Source: CAD feature listing. Evaluate the final solid. Frame: model axes, mm. Face numbers are marked on the shaded views. A direction names the side the tool comes from. Round coordinates to 2 decimals unless told otherwise and drop trailing zeros. Loops run counter-clockwise (first coordinate to the right, second up) from the corner with the lowest first, then second, coordinate; pieces in that order, holes last. Notation, with made-up numbers: M 21,44.5 L 30,44.5 A10 ccw 30,63.5 Z; hole C 43,8 d11. An arc over 180 degrees is marked long. Write each question's results on one line, items separated by ' | '. Start each with the question number.
1. Section A-A on x = -1.5. Output: boundary loops of the cut face in (y, z), and give its area (3 significant figures).
2. Section B-B on z = 7.5. Output: boundary loops of the cut face in (x, y).
3. Section D-D on y = -33.5. Output: boundary loops of the cut face in (x, z), and give its area (3 significant figures).
4. Section C-C on y = -7. Output: boundary loops of the cut face in (x, z), and give its area (3 significant figures).
5. Contact query for a flat-ended pin moving along its axis: pin 1 Ø1.6 at (x, z) = (12.5, -1.5) entering from -Y. Output: stop coordinate, or through.
6. Ray query, line 1 (X direction, y = -25, z = 17); line 2 (Z direction, x = 1, y = -25); line 3 (X direction, y = -21.5, z = -3). Return the intervals inside material, ascending.
7. Draft query along Z for the marked faces 1, 2 and 3. Return one class per face: released by +Z, released by -Z, zero draft, split by the parting line, or undercut.
8. Set-up query: the marked faces 4 and 5. Return all of +Z, -Z, +X, -X, +Y, -Y with unobstructed straight access to the full face (end or side cutting, diameter ignored); none if empty.
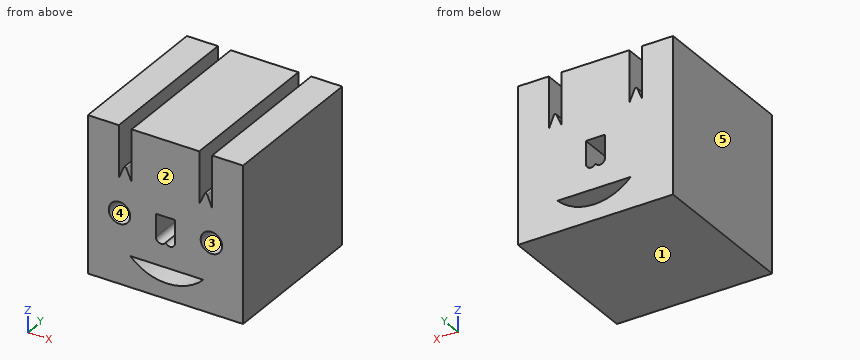
from build123d import *

# Parameters (mm, degrees)
F0_R     = 2.637924
F1_DEPTH = 38.1
F2_DEPTH = 19.05


with BuildPart() as f1:
    # F0 (on Front) → F1 (new body)
    with BuildSketch(Plane.XZ):
        with BuildLine():
            Line((-11.453714, 19.05), (-19.05, 19.05))
            Line((-19.05, 19.05), (-19.05, -19.05))
            Line((-19.05, -19.05), (19.05, -19.05))
            Line((19.05, -19.05), (19.05, 19.05))
            Line((19.05, 19.05), (11.453714, 19.05))
            Line((11.453714, 19.05), (11.453714, 6.35))
            Line((11.453714, 6.35), (10.227945, 9.297051))
            ThreePointArc((10.227945, 9.297051), (9.928561, 9.499715), (9.623805, 9.305221))
            Line((9.623805, 9.305221), (8.299793, 6.35))
            Line((8.299793, 6.35), (8.299793, 19.05))
            Line((8.299793, 19.05), (0, 19.05))
            Line((0, 19.05), (-8.299793, 19.05))
            Line((-8.299793, 19.05), (-8.299793, 6.35))
            Line((-8.299793, 6.35), (-9.623805, 9.305221))
            ThreePointArc((-9.623805, 9.305221), (-9.928561, 9.499715), (-10.227945, 9.297051))
            Line((-10.227945, 9.297051), (-11.453714, 6.35))
            Line((-11.453714, 6.35), (-11.453714, 19.05))
        make_face()
        with Locations((-11.287717, -1.99195)):
            Circle(F0_R, mode=Mode.SUBTRACT)
        with BuildLine():
            ThreePointArc((9.332039, -11.526389), (0.341904, -15.257474), (-8.648231, -11.526389))
            Line((-8.648231, -11.526389), (9.332039, -11.526389))
        make_face(mode=Mode.SUBTRACT)
        with BuildLine():
            Line((-2.361556, 0.645974), (0, 0.645974))
            Line((0, 0.645974), (2.361556, 0.645974))
            Line((2.361556, 0.645974), (2.361556, -4.915977))
            ThreePointArc((2.361556, -4.915977), (1.428174, -6.140554), (0, -5.565134))
            ThreePointArc((0, -5.565134), (-1.428174, -6.140554), (-2.361556, -4.915977))
            Line((-2.361556, -4.915977), (-2.361556, 0.645974))
        make_face(mode=Mode.SUBTRACT)
        with Locations((11.287717, -1.99195)):
            Circle(F0_R, mode=Mode.SUBTRACT)
    extrude(amount=F1_DEPTH)

    # F0 (on Front) → F2 (join)
    with BuildSketch(Plane.XZ):
        with Locations((-11.287717, -1.99195)):
            Circle(F0_R)
        with Locations((11.287717, -1.99195)):
            Circle(F0_R)
    extrude(amount=F2_DEPTH)


solid = f1.part
Taken from the geometry:
1) outline: M -38.1,-19.05 L 0,-19.05 L 0,-15.12 L -38.1,-15.12 Z; M -38.1,-11.53 L 0,-11.53 L 0,-6.12 L -38.1,-6.12 Z; M -38.1,0.65 L 0,0.65 L 0,19.05 L -38.1,19.05 Z | area: 1,060 mm^2
2) outline: M -19.05,-38.1 L -11.45,-38.1 L -11.45,0 L -19.05,0 Z; M -10.98,-38.1 L -8.82,-38.1 L -8.82,0 L -10.98,0 Z; M -8.3,-38.1 L 8.3,-38.1 L 8.3,0 L -8.3,0 Z; M 8.82,-38.1 L 10.98,-38.1 L 10.98,0 L 8.82,0 Z; M 11.45,-38.1 L 19.05,-38.1 L 19.05,0 L 11.45,0 Z
3) outline: M -19.05,-19.05 L 19.05,-19.05 L 19.05,19.05 L 11.45,19.05 L 11.45,6.35 L 10.23,9.3 A0.33 ccw 9.62,9.31 L 8.3,6.35 L 8.3,19.05 L -8.3,19.05 L -8.3,6.35 L -9.62,9.31 A0.33 ccw -10.23,9.3 L -11.45,6.35 L -11.45,19.05 L -19.05,19.05 Z; hole C -11.29,-1.99 d5.28; hole M -8.65,-11.53 A12.7 ccw 9.33,-11.53 Z; hole M -2.36,-4.92 A1.27 ccw 0,-5.57 A1.27 ccw 2.36,-4.92 L 2.36,0.65 L -2.36,0.65 Z; hole C 11.29,-1.99 d5.28 | area: 1,260 mm^2
4) outline: M -19.05,-19.05 L 19.05,-19.05 L 19.05,19.05 L 11.45,19.05 L 11.45,6.35 L 10.23,9.3 A0.33 ccw 9.62,9.31 L 8.3,6.35 L 8.3,19.05 L -8.3,19.05 L -8.3,6.35 L -9.62,9.31 A0.33 ccw -10.23,9.3 L -11.45,6.35 L -11.45,19.05 L -19.05,19.05 Z; hole M -8.65,-11.53 A12.7 ccw 9.33,-11.53 Z; hole M -2.36,-4.92 A1.27 ccw 0,-5.57 A1.27 ccw 2.36,-4.92 L 2.36,0.65 L -2.36,0.65 Z | area: 1,310 mm^2
5) pin 1: y = -19.05
6) line 1: -19.05 to -11.45, -8.3 to 8.3, 11.45 to 19.05 | line 2: -19.05 to -15.24, -11.53 to -6.18, 0.65 to 19.05 | line 3: -19.05 to -13.73, -8.85 to -2.36, 2.36 to 8.85, 13.73 to 19.05
7) face 1: released by -Z | face 2: zero draft | face 3: undercut
8) face 4: -Y | face 5: +Z, -Z, -X, +Y, -Y
